Design review of the part built by this model. Coordinates are the model's own, in mm. A direction names the side the tool comes from. Round coordinates to 2 decimals unless told otherwise and drop trailing zeros. Write each loop counter-clockwise with the first axis right and the second up, starting at its lowest first coordinate (ties: lowest second). Pieces come first, ordered by that corner, then holes. Notation, with made-up numbers: M 2.25,-11 L 18.25,-11 A22 ccw 18.25,5 Z; hole C 14.25,18 d6. An arc over 180 degrees is marked long. One line per question, with ' | ' between items. Start each with the question number.
Item 1: Machinability: for faces 1 (the face through (29, 1, 0)), 2 (the face through (25.019, 1, -2)), 3 (the face through (59, 1, -22.454)), which of the approach directions +Z, -Z, +X, -X, +Y, -Y give a long, thin tool a straight path to every point of the face, cutting with its end or side? Answer none if there is none.
Item 2: Add section A-A, the plane x = 50. State the section outline as (y, z) points.
Item 3: Add section C-C, the plane z = -23. State the section outline as (x, y) points, and give its area (3 significant figures).
Item 4: Draft analysis for pull direction X (two halves, no side actions). For faces 4 (the face through (31, 2.845, -12)), 5 (the face through (22.428, 1, -2)), 6 (the face through (33.945, 1.442, 0.043)), state which applies: released by +X, released by -X, zero draft, split by the parting line, or undercut.
Item 5: Add section D-D, the plane x = 34. State the section outline as (y, z) points, and give its area (3 significant figures).
Item 6: For L1, parallel to X at y = 0.35, z = -1; L2, parallel to X at y = 1.95, z = -0.5; L3, parallel to Z at x = 50.5, y = 2.15, list the stretches that pass through material, from the lowest coordinate up.
Item 7: Add section B-B, the plane y = 0.9. State the section outline as (x, z) points.
Item 8: Insertion check: pin 1 Ø1.4 at (y, z) = (2, -2.5) entering from +X; pin 2 Ø0.9 at (y, z) = (1, 0.5) entering from +X; pin 3 Ø1.4 at (x, y) = (58.5, 1) entering from +Z. Each pin has a flat end and moves straight along its axis. Give the tip position at first contact, or say it passes through.
```python
from build123d import *

# Parameters (mm, degrees)
BOSS_EXTRUDE1_DEPTH = 2.8448
FILLET1_R           = 12.7
CUT_EXTRUDE1_REACH  = 67.623
SKETCH2_W           = 2.5908
SKETCH2_H           = 4.1402
CUT_EXTRUDE2_REACH  = 67.623
SKETCH3_R           = 2.5908


with BuildPart() as part:
    # Sketch1 → Boss-Extrude1 (new body)
    with BuildSketch(Plane(origin=(0, 0, 0), x_dir=(1, 0, 0), z_dir=(0, 1, 0))):
        Polygon((0, 0), (0, 23.9014), (57.531, 25.3746), (57.531, 22.4536), (60.452, 22.4536), (59.7154, 0.5842), (56.7944, 0.5842), (56.7944, -2.3368), (48.1584, -2.3368), (33.9344, 0), align=None)
    extrude(amount=BOSS_EXTRUDE1_DEPTH)

    # Fillet1
    fillet1_edges = [part.edges().sort_by_distance(p)[0] for p in [
        (48.1584, 1.4224, 2.3368),
        (33.9344, 1.4224, 0),
    ]]
    fillet(fillet1_edges, radius=FILLET1_R)

    # Sketch2 → Cut-Extrude1 (cut, up to next)
    with BuildSketch(Plane(origin=(0, 2.8448, 0), x_dir=(1, 0, 0), z_dir=(0, 1, 0)), mode=Mode.PRIVATE) as cut_extrude1_sk1:
        with Locations((23.7236, 2.0701)):
            Rectangle(SKETCH2_W, SKETCH2_H)
    cut_extrude1_tool1 = extrude(cut_extrude1_sk1.sketch, amount=-CUT_EXTRUDE1_REACH, mode=Mode.PRIVATE) & part.part
    add(cut_extrude1_tool1.solids().sort_by_distance((23.7236, 2.8448, -2.0701))[0], mode=Mode.SUBTRACT)

    # Sketch3 → Cut-Extrude2 (cut, up to next)
    with BuildSketch(Plane(origin=(0, 2.8448, 0), x_dir=(1, 0, 0), z_dir=(0, 1, 0)), mode=Mode.PRIVATE) as cut_extrude2_sk1:
        with Locations(Location((50.8508, 18.7198, 0), (0, 0, 270))):
            Circle(SKETCH3_R)
    cut_extrude2_tool1 = extrude(cut_extrude2_sk1.sketch, amount=-CUT_EXTRUDE2_REACH, mode=Mode.PRIVATE) & part.part
    add(cut_extrude2_tool1.solids().sort_by_distance((50.8508, 2.8448, -18.7198))[0], mode=Mode.SUBTRACT)


solid = part.part
```
Computed values:
1) face 1: +Z, -X, +Y, -Y | face 2: +Z, +Y, -Y | face 3: -Z, +X, +Y, -Y
2) outline: M 0,-25.18 L 2.84,-25.18 L 2.84,-21.17 L 0,-21.17 Z; M 0,-16.27 L 2.84,-16.27 L 2.84,2.34 L 0,2.34 Z
3) outline: M 0,0 L 57.53,0 L 57.53,2.84 L 0,2.84 Z | area: 164 mm^2
4) face 4: zero draft | face 5: undercut | face 6: released by -X
5) outline: M 0,-24.77 L 2.84,-24.77 L 2.84,0.05 L 0,0.05 Z | area: 70.6 mm^2
6) L1: x = 0 to 22.43, 25.02 to 59.73 | L2: x = 0 to 22.43, 25.02 to 56.79 | L3: z = -25.19 to -21.29, -16.15 to 2.34
7) outline: M 0,-23.9 L 57.53,-25.37 L 57.53,-22.45 L 60.45,-22.45 L 59.72,-0.58 L 56.79,-0.58 L 56.79,2.34 L 49.19,2.34 A12.7 ccw 47.14,2.17 L 34.96,0.17 A12.7 cw 32.9,0 L 25.02,0 L 25.02,-4.14 L 22.43,-4.14 L 22.43,0 L 0,0 Z; hole C 50.85,-18.72 d5.18
8) pin 1: stops at x = 59.8 | pin 2: stops at x = 56.79 | pin 3: stops at z = -0.58
